Read the model definition and answer for the solid it produces. Units are mm, in the model's axes. A direction names the side the tool comes from. Coordinates: 2 decimals unless noted, no trailing zeros. Order: outer loops, then holes, each group sorted by start corner. A loop starts at its lowest first (then second) coordinate and runs counter-clockwise, first axis right, second up.
from build123d import *

# Parameters (mm, degrees)
F0_W     = 40
F0_H     = 40
F1_DEPTH = 2
F2_W     = 2
F2_H     = 40
F3_DEPTH = 2
F4_W     = 2
F4_H     = 40
F5_DEPTH = 2


with BuildPart() as f1:
    # F0 (on Top) → F1 (new body)
    with BuildSketch(Plane.XY):
        Rectangle(F0_W, F0_H)
    extrude(amount=F1_DEPTH)

    # F2 (on face) → F3 (join)
    with BuildSketch(Plane.YZ.offset(20)):
        with Locations((19, -20)):
            Rectangle(F2_W, F2_H)
        with Locations((-19, -20)):
            Rectangle(F2_W, F2_H)
    extrude(amount=-F3_DEPTH)

    # F4 (on face) → F5 (join)
    with BuildSketch(Plane(origin=(-20, 0, 0), x_dir=(0, -1, 0), z_dir=(-1, 0, 0))):
        with Locations((-19, -20)):
            Rectangle(F4_W, F4_H)
        with Locations((19, -20)):
            Rectangle(F4_W, F4_H)
    extrude(amount=-F5_DEPTH)


solid = f1.part
Q1. Determine the mould class of faces 4 (the flat face through (18, -19, -20)), 5 (the flat face through (-18, -19, -20)), 6 (the flat face through (20, 0, 1)), 7 (the flat face through (0, -20, 1)) for opening direction X: +X half, -X half, draft (parallel to the pull), parting line (faces both ways), or undercut.
Q2. The part is cut by section B-B, the plane x = 14. Determine the outline of the cut face in (y, z), then the cut area to 3 significant figures.
Q3. The part is cut by section A-A, the plane z = -7.5. Determine the outline of the cut face in (x, y), then the cut area to 3 significant figures.
Q4. Which of the six approach directions +Z, -Z, +X, -X, +Y, -Y give full straight-line access (tool end or side, diameter ignored) to faces 1 (the flat face through (-19, 18, -20)), 2 (the flat face through (0, 0, 2)), 3 (the flat face through (-18, 19, -20))?
Q5. A straight line is drawn through the part: L1, parallel to Z at x = 8, y = 15. Find the intervals that lie inside material, in ascending order.
Computed values:
1. face 4: undercut
1. face 5: undercut
1. face 6: +X half
1. face 7: draft
2. outline: (-20, 0) - (20, 0) - (20, 2) - (-20, 2) - close
2. area: 80.0 mm2
3. outline: (-20, -20) - (-18, -20) - (-18, -18) - (-20, -18) - close; (-20, 18) - (-18, 18) - (-18, 20) - (-20, 20) - close; (18, -20) - (20, -20) - (20, -18) - (18, -18) - close; (18, 18) - (20, 18) - (20, 20) - (18, 20) - close
3. area: 16.0 mm2
4. face 1: -Z, +X, -X
4. face 2: +Z, +X, -X, +Y, -Y
4. face 3: -Z, +Y, -Y
5. L1: z = 0 to 2
